from build123d import *

# Parameters (mm, degrees)
F0_W      = 75
F0_H      = 75
F1_DEPTH  = 3
F2_R      = 2
F3_DEPTH  = 2
F4_R      = 1.25
F5_DEPTH  = 1.001
F6_W      = 15
F6_H      = 1.5
F7_DEPTH  = 20
F8_W      = 12
F8_H      = 1.5
F9_DEPTH  = 20
F10_R     = 1.25
F11_DEPTH = 23.001


with BuildPart() as f1:
    # F0 (on Top) → F1 (new body)
    with BuildSketch(Plane.XY):
        Rectangle(F0_W, F0_H)
    extrude(amount=F1_DEPTH)

    # F2 (on face) → F3 (cut)
    with BuildSketch(Plane.XY.offset(3)):
        with Locations((31.5, -20)):
            Circle(F2_R)
        with Locations((20, -31.5)):
            Circle(F2_R)
        with Locations((31.5, 20)):
            Circle(F2_R)
        with Locations((20, 31.5)):
            Circle(F2_R)
        with Locations((-20, 31.5)):
            Circle(F2_R)
        with Locations((-31.5, 20)):
            Circle(F2_R)
        with Locations((-20, -31.5)):
            Circle(F2_R)
        with Locations((-31.5, -20)):
            Circle(F2_R)
    extrude(amount=-F3_DEPTH, mode=Mode.SUBTRACT)

    # F4 (on face) → F5 (cut, through all)
    with BuildSketch(Plane.XY.offset(1)):
        with Locations((-31.5, 20)):
            Circle(F4_R)
        with Locations((-20, 31.5)):
            Circle(F4_R)
        with Locations((20, 31.5)):
            Circle(F4_R)
        with Locations((31.5, 20)):
            Circle(F4_R)
        with Locations((-31.5, -20)):
            Circle(F4_R)
        with Locations((31.5, -20)):
            Circle(F4_R)
        with Locations((20, -31.5)):
            Circle(F4_R)
        with Locations((-20, -31.5)):
            Circle(F4_R)
    extrude(amount=-F5_DEPTH, mode=Mode.SUBTRACT)

    # F6 (on face) → F7 (join)
    with BuildSketch(Plane.XY.offset(3)):
        with Locations((0, -23.75)):
            Rectangle(F6_W, F6_H)
        with Locations((0, 23.75)):
            Rectangle(F6_W, F6_H)
    extrude(amount=F7_DEPTH)

    # F8 (on face) → F9 (join)
    with BuildSketch(Plane.XY.offset(3)):
        with Locations((0, -35.75)):
            Rectangle(F8_W, F8_H)
        with Locations((0, 35.75)):
            Rectangle(F8_W, F8_H)
    extrude(amount=F9_DEPTH)

    # F10 (on face) → F11 (cut, through all)
    with BuildSketch(Plane(origin=(0, 0, 0), x_dir=(1, 0, 0), z_dir=(0, 0, -1))):
        Polygon((37.5, 37.5), (4.855387, 37.5), (37.5, 7.5), align=None)
        Polygon((37.5, 37.5), (4.855387, 37.5), (37.5, 7.5), align=None)
        with Locations((31.5, 20)):
            Circle(F10_R, mode=Mode.SUBTRACT)
        with Locations((20, 31.5)):
            Circle(F10_R, mode=Mode.SUBTRACT)
    extrude(amount=-F11_DEPTH, mode=Mode.SUBTRACT)


solid = f1.part
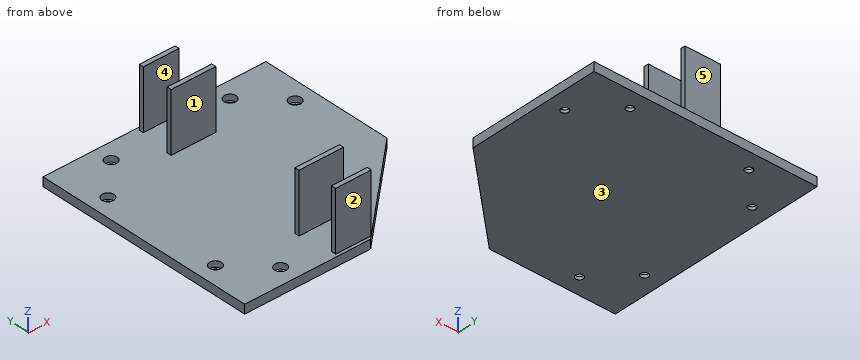
Read the model definition and answer for the solid it produces. Units are mm, in the model's axes. Face numbers are marked on the shaded views. A direction names the side the tool comes from. Give positions to 0.01 mm unless a question says otherwise; leave off trailing zeros. Write each loop counter-clockwise with the first axis right and the second up, starting at its lowest first coordinate (ties: lowest second). Pieces come first, ordered by that corner, then holes. Notation, with made-up numbers: (-27, 1.5) -> (-10, 1.5) arc R15 ccw to (-10, 18.5) -> close; hole circle Ø10 at (32.25, -39). An arc over 180 degrees is marked (long way). Answer as a JSON object with one key per item and string values. Group by question number.
1) Each of these flat-tipped pins is pushed along its axis until it touches: P1, Ø1.6, axis at y = 23.5, z = 9, coming from the -X side; P2, Ø1.6, axis at y = -35.5, z = 8, coming from the +X side; P3, Ø3.5, axis at x = -1.5, z = 9.5, coming from the -Y side. Where does it stop, or does it pass through?
2) Find section A-A (x = -20). Write down the section's boundary in (y, z), and give its area (3 significant figures).
3) Consider L1, parallel to Y at x = 2, z = 14.5; L2, parallel to Y at x = -20, z = 2.1; L3, parallel to Z at x = -29.5, y = 14.5. Determine where each line is inside the solid, lowest interval first. Write a range as from..to.
4) Find section B-B (y = 31.5). Write down the section's boundary in (x, z), and give its area (3 significant figures).
5) The mould has two halves that part along Y. Classify the marked faces 1, 2 and 3: +Y half, -Y half, draft (parallel to the pull), parting line (faces both ways), or undercut.
6) A tool of negligible diameter and unlimited length cuts with its end or side. For the marked faces 4 and 5, from which of +Z, -Z, +X, -X, +Y, -Y can it reach the whole face along a straight path? Write none if from no direction.
7) Find section C-C (z = 4.25). Write down the section's boundary in (x, y), and give its area (3 significant figures).
8) Find section D-D (y = -31.5). Write down the section's boundary in (x, z).
Values follow:
{
 "1": {"P1": "stops at x = -7.5", "P2": "stops at x = 6", "P3": "stops at y = -36.5"},
 "2": {"outline": "(-37.5, 0) -> (-32.75, 0) -> (-32.75, 1) -> (-33.5, 1) -> (-33.5, 3) -> (-37.5, 3) -> close; (-30.25, 0) -> (30.25, 0) -> (30.25, 1) -> (29.5, 1) -> (29.5, 3) -> (-29.5, 3) -> (-29.5, 1) -> (-30.25, 1) -> close; (32.75, 0) -> (37.5, 0) -> (37.5, 3) -> (33.5, 3) -> (33.5, 1) -> (32.75, 1) -> close", "area": "204 mm2"},
 "3": {"L1": "y = -36.5..-35, -24.5..-23, 23..24.5, 35..36.5", "L2": "y = -37.5..-33.5, -29.5..29.5, 33.5..37.5", "L3": "z = 0..3"},
 "4": {"outline": "(-37.5, 0) -> (-21.25, 0) -> (-21.25, 1) -> (-22, 1) -> (-22, 3) -> (-37.5, 3) -> close; (-18.75, 0) -> (18.75, 0) -> (18.75, 1) -> (18, 1) -> (18, 3) -> (-18, 3) -> (-18, 1) -> (-18.75, 1) -> close; (21.25, 0) -> (37.5, 0) -> (37.5, 3) -> (22, 3) -> (22, 1) -> (21.25, 1) -> close", "area": "204 mm2"},
 "5": {"face 1": "undercut", "face 2": "-Y half", "face 3": "draft"},
 "6": {"face 4": "+Z, +X, -X", "face 5": "+Z, +X, -X, +Y"},
 "7": {"outline": "(-7.5, -24.5) -> (7.5, -24.5) -> (7.5, -23) -> (-7.5, -23) -> close; (-7.5, 23) -> (7.5, 23) -> (7.5, 24.5) -> (-7.5, 24.5) -> close; (-6, -36.5) -> (5.94, -36.5) -> (6, -36.45) -> (6, -35) -> (-6, -35) -> close; (-6, 35) -> (6, 35) -> (6, 36.5) -> (-6, 36.5) -> close", "area": "81.0 mm2"},
 "8": {"outline": "(-37.5, 0) -> (-21.25, 0) -> (-21.25, 1) -> (-22, 1) -> (-22, 3) -> (-37.5, 3) -> close; (-18.75, 0) -> (11.38, 0) -> (11.38, 3) -> (-18, 3) -> (-18, 1) -> (-18.75, 1) -> close"}
}
